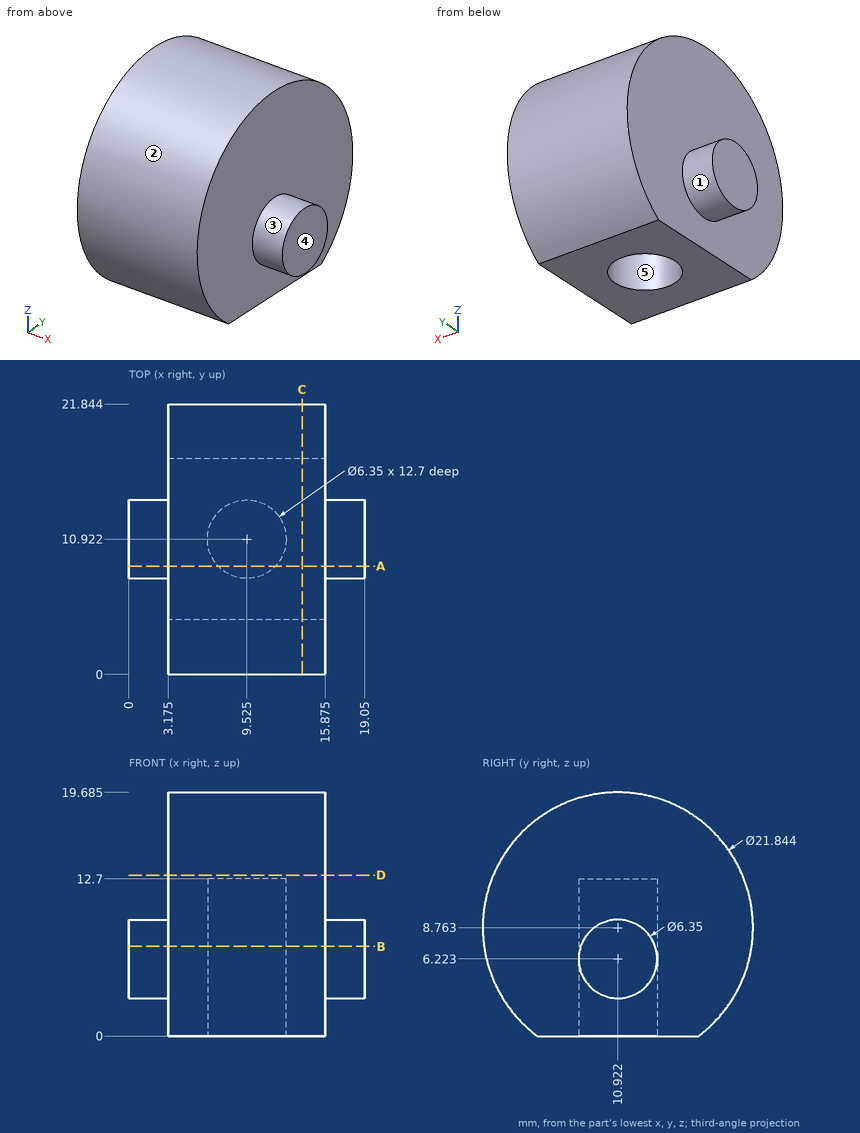
Geometry check sheet. Reference: drawing and pictorial views, mm from the part's lowest x, y, z. A direction names the side the tool comes from. Give positions to 0.01 mm unless a question says otherwise; leave off trailing zeros. Loops run counter-clockwise (first coordinate to the right, second up) from the corner with the lowest first, then second, coordinate; pieces in that order, holes last.
1. Section check C-C, the plane x = 14. Enter the section's corners in (y, z).
2. Section check D-D, the plane z = 13. Enter the section's corners in (x, y) (3 decimals).
3. Thickness scan on line 1 (Y direction, x = 14, z = 8.5); line 2 (X direction, y = 2.75, z = 4) (3 decimals); line 3 (X direction, y = 12.5, z = 6.5). Record the ranges inside material, lowest first.
4. Mould release check, pull along Y, two halves, no side actions. Record for the marked faces 3, 4 and 5: released by +Y, released by -Y, zero draft, split by the parting line, or undercut.
5. Section check B-B, the plane z = 7.25. Enter the section's corners in (x, y) (3 decimals).
6. Section check A-A, the plane y = 8.75. Enter the section's corners in (x, z) (3 decimals).
7. Set-up check for the marked faces 1 and 2: record each of +Z, -Z, +X, -X, +Y, -Y from which the full face is reachable in a straight line by a thin tool's end or side.
8. Go/stop test with flat-tipped pins: pin 1 Ø1 at (x, y) = (8, 7.5) entering from +Z; pin 2 Ø2 at (x, z) = (9.5, 5.5) entering from +Y; pin 3 Ø5.5 at (x, y) = (9.525, 10.922) entering from -Z. Record where each tip stops, or that it passes through.
Geometry says:
1. outline: (4.4, 0) - (17.44, 0) arc R10.92 ccw (long way) to start
2. outline: (3.175, 0.855) - (15.875, 0.855) - (15.875, 20.989) - (3.175, 20.989) - close
3. line 1: y = 0 to 21.84
3. line 2: x = 3.175 to 15.875
3. line 3: x = 0 to 6.77, 12.28 to 19.05
4. face 3: split by the parting line
4. face 4: zero draft
4. face 5: undercut
5. outline: (0, 7.918) - (3.175, 7.918) - (3.175, 0.105) - (15.875, 0.105) - (15.875, 7.918) - (19.05, 7.918) - (19.05, 13.926) - (15.875, 13.926) - (15.875, 21.739) - (3.175, 21.739) - (3.175, 13.926) - (0, 13.926) - close; hole circle Ø6.35 at (9.525, 10.922)
6. outline: (0, 3.907) - (3.175, 3.907) - (3.175, 0) - (7.209, 0) - (7.209, 12.7) - (11.841, 12.7) - (11.841, 0) - (15.875, 0) - (15.875, 3.907) - (19.05, 3.907) - (19.05, 8.539) - (15.875, 8.539) - (15.875, 19.467) - (3.175, 19.467) - (3.175, 8.539) - (0, 8.539) - close
7. face 1: -X
7. face 2: +X, -X
8. pin 1: stops at z = 19.29
8. pin 2: stops at y = 21.61
8. pin 3: stops at z = 12.7
